Input: part model. Units: mm. Frame: model coordinates. Face numbers are marked on the shaded views. A direction names the side the tool comes from. Give positions to 0.01 mm unless a question says otherwise; leave off trailing zeros. Loops run counter-clockwise (first coordinate to the right, second up) from the corner with the lowest first, then second, coordinate; pieces in that order, holes last. Notation, with made-up numbers: M 40,72.5 L 84,72.5 A20 ccw 84,77.5 Z; hole C 23.25,-3 d2. An arc over 180 degrees is marked long. Answer as a JSON object with one key per item and string values. Group by question number.
1) Draft query along Y for the marked faces 3, 4 and 5. Return one class per face: +Y half, -Y half, draft (parallel to the pull), parting line (faces both ways), or undercut.
2) Section query C-C on z = 6.5. Return loops of the section in (x, y), plus the area to 3 significant figures.
3) Section query A-A on x = 0. Return loops of the section in (y, z).
4) Ray query, L1, parallel to Y at x = 0, z = 3; L2, parallel to Y at x = 0, z = 8.7; L3, parallel to X at y = 1.75, z = 3.25. Return the intervals inside material, ascending.
5) Access query for the marked faces 1 and 2. Directions: +Z, -Z, +X, -X, +Y, -Y. A direction counts if a zero-diameter tool reaches every point of the face in a straight line with its end or side. Return the directions, or none.
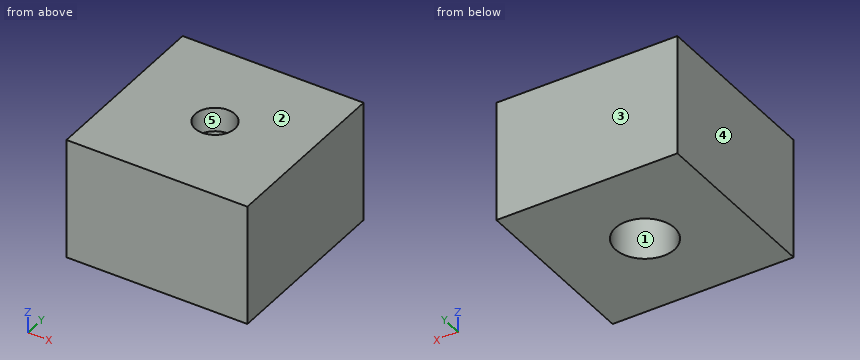
from build123d import *

# Parameters (mm, degrees)
SKETCH1_W           = 15
SKETCH1_H           = 15
SKETCH1_R           = 5
SKETCH1_R_2         = 2.45
SKETCH1_R_3         = 1.65
BOSS_EXTRUDE4_DEPTH = 10
SKETCH1_9_R         = 2.45
SKETCH1_9_R_2       = 1.65
CUT_EXTRUDE3_DEPTH  = 8


with BuildPart() as part:
    # Sketch1 → Boss-Extrude4 (new body)
    # profile 1 of 3: a face of its own
    with BuildSketch(Plane.XY):
        Rectangle(SKETCH1_W, SKETCH1_H)
        Circle(SKETCH1_R, mode=Mode.SUBTRACT)
    # profile 2 of 3: a face of its own
    with BuildSketch(Plane.XY):
        Circle(SKETCH1_R)
        Circle(SKETCH1_R_2, mode=Mode.SUBTRACT)
    # profile 3 of 3: a face of its own
    with BuildSketch(Plane.XY):
        Circle(SKETCH1_R_2)
        Circle(SKETCH1_R_3, mode=Mode.SUBTRACT)
    extrude(amount=BOSS_EXTRUDE4_DEPTH)

    # Sketch1_9 → Cut-Extrude3 (cut)
    with BuildSketch(Plane.XY):
        Circle(SKETCH1_9_R)
        Circle(SKETCH1_9_R_2, mode=Mode.SUBTRACT)
    extrude(amount=CUT_EXTRUDE3_DEPTH, mode=Mode.SUBTRACT)


solid = part.part
Output:
{
 "1": {"face 3": "+Y half", "face 4": "draft", "face 5": "undercut"},
 "2": {"outline": "M -7.5,-7.5 L 7.5,-7.5 L 7.5,7.5 L -7.5,7.5 Z; hole C 0,0 d4.9", "area": "206 mm^2"},
 "3": {"outline": "M -7.5,0 L -2.45,0 L -2.45,8 L -1.65,8 L -1.65,10 L -7.5,10 Z; M 1.65,8 L 2.45,8 L 2.45,0 L 7.5,0 L 7.5,10 L 1.65,10 Z"},
 "4": {"L1": "y = -7.5 to -2.45, 2.45 to 7.5", "L2": "y = -7.5 to -1.65, 1.65 to 7.5", "L3": "x = -7.5 to -1.71, 1.71 to 7.5"},
 "5": {"face 1": "-Z", "face 2": "+Z, +X, -X, +Y, -Y"}
}
